Design review of the part built by this model. Coordinates are the model's own, in mm. A direction names the side the tool comes from. Coordinates: 2 decimals unless noted, no trailing zeros. Loops run counter-clockwise (first coordinate to the right, second up) from the corner with the lowest first, then second, coordinate; pieces in that order, holes last. Notation, with made-up numbers: (74, -19) - (132, -19) arc R15 ccw to (132, -10) - close; hole circle Ø11 at (-40, 87). An arc over 180 degrees is marked (long way). Answer in a Markdown table with one row per item. Add a question column.
(1) We need section B-B, the plane y = 13. Write out the cut boundary in (x, z).
(2) For faces 1 (the face through (22, -6, -26.65)), 2 (the face through (-2.5, 11, 0)), 3 (the face through (-1.5, -20, 0)), list the 3-axis set-ups (+Z, -Z, +X, -X, +Y, -Y) from which the entire face can be reached by the end or side of a thin tool; tool diameter is ignored.
(3) Clearance check with flat-ended pins moving along their axes: pin 1 (1 mm diameter, centred on y = 4.5, z = -16.5, fed in from -X); pin 2 (3 mm diameter, centred on y = 4, z = -21.5, fed in from +X); pin 3 (5.5 mm diameter, centred on x = -12.5, z = 0, fed in from +Y). State where each tip first meets the part, or that it passes through.
(4) To check wall thickness, follow L1, parallel to Z at x = 11.4, y = 18.15; L2, parallel to X at y = 0.5, z = 0; L3, parallel to Z at x = 10, y = 7. State the ranges of each line that lie inside material, in increasing order. Write a range as [from, to].
(5) We need section A-A, the plane z = 0. Give the number of separate pieces and of enclosed holes in the cut face, plus the area to 3 significant figures.
(6) The part is to be moulded in two halves that separate along Z. For faces 4 (the face through (-28, 3, 0)), 5 (the face through (-6.54, 1.52, -18.01)), 6 (the face through (27.07, -19.484, -28.365)), say which applies: released by +Z, released by -Z, zero draft, split by the parting line, or undercut.
from build123d import *

# Parameters (mm, degrees)
SKETCH1_W            = 104.6
SKETCH1_H            = 57.3
BOSS_EXTRUDE1_DEPTH  = 3
SKETCH3_W            = 3
SKETCH3_H            = 57.3
BOSS_EXTRUDE3_DEPTH  = 40
M3_CLEARANCE_HOLE1_D = 3.4
BOSS_EXTRUDE4_DEPTH  = 2
SKETCH11_R           = 12.5
CUT_EXTRUDE1_DEPTH   = 72.806075648
M3_CLEARANCE_HOLE3_D = 3.4
SKETCH14_R           = 1.7
CUT_EXTRUDE2_DEPTH   = 74.51947021
BOSS_EXTRUDE5_START  = 16
SKETCH16_W           = 50.8
SKETCH16_H           = 57.3
SKETCH16_R           = 12.5
SKETCH16_R_2         = 1.7
BOSS_EXTRUDE5_DEPTH  = 16
SKETCH17_W           = 50.8
SKETCH17_H           = 53.3
CUT_EXTRUDE3_DEPTH   = 16
SKETCH18_W           = 57.3
SKETCH18_H           = 16
BOSS_EXTRUDE6_DEPTH  = 4
FILLET1_R            = 1


with BuildPart() as part:
    # Sketch1 → Boss-Extrude1 (new body)
    with BuildSketch(Plane(origin=(0, 0, 0), x_dir=(1, 0, 0), z_dir=(0, 1, 0))):
        Rectangle(SKETCH1_W, SKETCH1_H)
    extrude(amount=BOSS_EXTRUDE1_DEPTH)

    # Sketch3 → Boss-Extrude3 (add)
    with BuildSketch(Plane.XZ):
        Rectangle(SKETCH3_W, SKETCH3_H)
    extrude(amount=BOSS_EXTRUDE3_DEPTH)

    # M3 Clearance Hole1 (through all)
    with Locations(Plane(origin=(0, 0, 0), x_dir=(-1, 0, 0), z_dir=(0, -1, 0))):
        with Locations((-11.4, -15.5), (-42.4, 15.5), (-42.4, -15.5), (-11.4, 15.5)):
            Hole(M3_CLEARANCE_HOLE1_D / 2)

    # Sketch10 → Boss-Extrude4 (add)
    with BuildSketch(Plane.XY.offset(28.65)):
        Polygon((-52.3, 0), (-1.5, -40), (-1.5, 0), align=None)
        Polygon((1.5, -40), (52.3, 0), (1.5, 0), align=None)
    boss_extrude4 = extrude(amount=-BOSS_EXTRUDE4_DEPTH)

    # Mirror1: Boss-Extrude4 across plane
    add(boss_extrude4.mirror(Plane(origin=(0, 0, 0), x_dir=(1, 0, 0), z_dir=(0, 0, -1))))

    # Sketch11 → Cut-Extrude1 (cut, through all)
    with BuildSketch(Plane.XZ):
        with Locations(Location((26.9, 0, 0), (0, 0, 270))):
            Circle(SKETCH11_R)
    extrude(amount=-CUT_EXTRUDE1_DEPTH, mode=Mode.SUBTRACT)

    # M3 Clearance Hole3 (through all)
    with Locations(Plane(origin=(0, 0, 0), x_dir=(-1, 0, 0), z_dir=(0, -1, 0))):
        with Locations((45.638207547, -17.5), (8.161792453, 17.5), (8.161792453, -17.5), (45.638207547, 17.5)):
            Hole(M3_CLEARANCE_HOLE3_D / 2)

    # Sketch14 → Cut-Extrude2 (cut, through all)
    with BuildSketch(Plane(origin=(0, 3, 0), x_dir=(1, 0, 0), z_dir=(0, 1, 0))):
        with Locations(Location((-12.5, -4e-09, 0), (0, 0, 270))):
            Circle(SKETCH14_R)
        with Locations(Location((-22.5, -4e-09, 0), (0, 0, 270))):
            Circle(SKETCH14_R)
    extrude(amount=-CUT_EXTRUDE2_DEPTH, mode=Mode.SUBTRACT)

    # Sketch16 → Boss-Extrude5 (add)
    with BuildSketch(Plane(origin=(0, 3, 0), x_dir=(1, 0, 0), z_dir=(0, 1, 0)).offset(BOSS_EXTRUDE5_START)):
        with Locations((26.9, 0)):
            Rectangle(SKETCH16_W, SKETCH16_H)
        with Locations(Location((26.9, 0, 0), (0, 0, 90))):
            Circle(SKETCH16_R, mode=Mode.SUBTRACT)
        with Locations(Location((42.4, 15.5, 0), (0, 0, 90))):
            Circle(SKETCH16_R_2, mode=Mode.SUBTRACT)
        with Locations(Location((42.4, -15.5, 0), (0, 0, 90))):
            Circle(SKETCH16_R_2, mode=Mode.SUBTRACT)
        with Locations(Location((11.4, -15.5, 0), (0, 0, 90))):
            Circle(SKETCH16_R_2, mode=Mode.SUBTRACT)
        with Locations(Location((11.4, 15.5, 0), (0, 0, 90))):
            Circle(SKETCH16_R_2, mode=Mode.SUBTRACT)
    extrude(amount=-BOSS_EXTRUDE5_DEPTH)

    # Sketch17 → Cut-Extrude3 (cut)
    with BuildSketch(Plane.XZ):
        with Locations((26.9, 0)):
            Rectangle(SKETCH17_W, SKETCH17_H)
    extrude(amount=-CUT_EXTRUDE3_DEPTH, mode=Mode.SUBTRACT)

    # Sketch18 → Boss-Extrude6 (add)
    with BuildSketch(Plane.ZY.offset(-1.5)):
        with Locations((0, 11)):
            Rectangle(SKETCH18_W, SKETCH18_H)
    extrude(amount=BOSS_EXTRUDE6_DEPTH)

    # Fillet1
    fillet1_edges = [part.edges().sort_by_distance(p)[0] for p in [
        (52.3, 19, 0),
        (24.9, 19, -28.65),
        (24.9, 19, 28.65),
        (26.9, 19, 12.5),
        (1.5, 16, 0),
        (26.9, 16, 26.65),
        (26.9, 16, -26.65),
        (-27.4, 3, 28.65),
        (0, -40, -28.65),
        (-27.4, 3, -28.65),
        (-2.5, 11, -28.65),
        (-2.5, 3, 0),
        (-2.5, 11, 28.65),
        (-2.5, 19, 0),
        (0, -40, 28.65),
        (-1.5, 0, 0),
        (-26.9, 0, 26.65),
        (-1.5, -20, 26.65),
        (-26.9, -20, 28.65),
        (1.5, -12, 26.65),
        (26.9, -20, 28.65),
        (-26.9, -20, -28.65),
        (-26.9, 0, -26.65),
        (-1.5, -20, -26.65),
        (52.3, 9.5, 28.65),
        (-52.3, 1.5, 28.65),
        (26.9, -20, -28.65),
        (-52.3, 1.5, -28.65),
        (1.5, -12, -26.65),
        (52.3, 9.5, -28.65),
    ]]
    fillet(fillet1_edges, radius=FILLET1_R)


solid = part.part
Responses:
| question | item | result |
|---|---|---|
| 1 | outline | (-2.5, -27.65) arc R1 ccw to (-1.5, -28.65) - (51.3, -28.65) arc R1 ccw to (52.3, -27.65) - (52.3, -26.65) - (2.5, -26.65) arc R1 cw to (1.5, -25.65) - (1.5, 25.65) arc R1 cw to (2.5, 26.65) - (52.3, 26.65) - (52.3, 27.65) arc R1 ccw to (51.3, 28.65) - (-1.5, 28.65) arc R1 ccw to (-2.5, 27.65) - close |
| 2 | face 1 | +X, -Y |
| 2 | face 2 | +Z, -Z, -X, +Y |
| 2 | face 3 | -X, -Y |
| 3 | pin 1 | stops at x = -2.5 |
| 3 | pin 2 | stops at x = 1.5 |
| 3 | pin 3 | stops at y = 3 |
| 4 | L1 | z = [-28.64, -17.2], [-13.8, 13.8], [17.2, 28.64] |
| 4 | L2 | x = [-52.3, -24.2], [-20.8, -14.2], [-10.8, 1.5] |
| 4 | L3 | z = [-28.65, -26.65], [26.65, 28.65] |
| 5 | separate pieces | 4 |
| 5 | enclosed holes | 0 |
| 5 | area | 402 mm2 |
| 6 | face 4 | zero draft |
| 6 | face 5 | undercut |
| 6 | face 6 | released by -Z |
